Model file for the job. Use its own axes, mm. A direction names the side the tool comes from. Give positions to 0.01 mm unless a question says otherwise; leave off trailing zeros. Order: outer loops, then holes, each group sorted by start corner. A loop starts at its lowest first (then second) coordinate and runs counter-clockwise, first axis right, second up. Notation, with made-up numbers: (6, 35) - (10, 35) arc R6 cw to (10, 45) - close; hole circle Ø9 at (43.5, 52.5). An arc over 180 degrees is marked (long way). Use CSV: the item, a comma, the result in double quotes. Start each with the question number.
(1) Band-saw the part on B-B, the plane x = 0. Give the cut face in (y, z), then the cut area to 3 significant figures.
(2) Probe L1, parallel to Z at x = 5.2, y = 0 (3 decimals); L2, parallel to Z at x = 4, y = -1.25; L3, parallel to Y at x = 5.3, z = 7 (3 decimals). List the from-to ranges inside material, lowest first.
(3) Band-saw the part on C-C, the plane z = 11.5. Give the cut face in (x, y), then the cut area to 3 significant figures.
(4) Drop flat-ended pins along their axis: pin 1 Ø1 at (y, z) = (6, 15.5) entering from +X; pin 2 Ø10 at (y, z) = (-4, 25.5) entering from +X; pin 3 Ø8 at (x, z) = (-5, 24.5) entering from -Y; pin 4 Ø5 at (y, z) = (4, 29) entering from +X. Give the stop position or say it passes through.
(5) Pull direction X, two halves, no side cores. Call faces 1 (the cylindrical face through (4.57, -7.167, 16.769)), 2 (the cylindrical face through (-3.686, -0.162, 8.874)), 3 (the flat face through (3, 0, 34)): +X half, -X half, draft (parallel to the pull), parting line (faces both ways), or undercut.
(6) Band-saw the part on A-A, the plane y = 0. Give the cut face in (x, z) (3 decimals).
(7) Band-saw the part on D-D, the plane z = 27. Give the cut face in (x, y) (3 decimals), then the cut area to 3 significant figures.
(8) Tool access for faces 4 (the flat face through (1.815, 0, 29)), 5 (the flat face through (3.4, 1.9, 0)), 6 (the cylindrical face through (5.92, -1.36, 7.43)), 7 (the flat face through (0, 0, 18)): list every direction of +Z, -Z, +X, -X, +Y, -Y with a clear straight run to the whole face (end or side of a thin tool).
Autodesk Inventor part; units mm, degrees
ref_plane "Work Plane2" through (6, -1.3086, 34) normal (1, 0, 0) x (0, -1, 0)
ref_plane "YZ Plane" through (0, 0, 0) normal (1, 0, 0) x (0, 1, 0)
ref_plane "XZ Plane" through (0, 0, 0) normal (0, 1, 0) x (-1, 0, 0)
sketch "Sketch1" plane through (0, 0, 0) normal (0, 0, 1) x (1, 0, 0)
  circle A0 centre (0, 0) radius 8.5
  circle A1 centre (0, 0) radius 3.69
  dimension "d0" = 17
  dimension "d3" = 7.38
  dimension "d20" = 4.81
extrude "Extrusion2" add sketch "Sketch1" along normal blind 18
sketch "Sketch2" plane through (0, 0, 18) normal (0, 0, 1) x (1, 0, 0)
  circle A0 centre (0, 0) radius 8.5
  circle A1 centre (0, 0) radius 8.5
extrude "Extrusion3" add sketch "Sketch2" along normal blind 4
sketch "Sketch3" plane through (0, 0, 22) normal (0, 0, 1) x (1, 0, 0)
  arc A0 (1.815, 2.6173) -> (1.815, -2.6173) centre (0, 0) ccw
  circle A1 centre (0, 0) radius 8.5
  line L0 (1.815, 2.6173) -> (1.815, -2.6173)
  circle A2 centre (0, 0) radius 8.5
  dimension "d8" = 6.37
  dimension "d11" = 5
  dimension "d12" = 1.815
extrude "Extrusion4" add sketch "Sketch3" along normal blind 12
ref_plane "Work Plane2" through (6, -1.3086, 34) normal (1, 0, 0) x (0, -1, 0)
ref_plane "Work Plane1" through (1.815, -1.3086, 34) normal (1, 0, 0) x (0, -1, 0)
sketch "Sketch4" plane through (6, -1.3086, 34) normal (1, 0, 0) x (0, -1, 0)
  circle A0 centre (-1.3086, 7) radius 1.425
  circle A1 centre (-1.3086, 27) radius 1.425
  line L0 (-9.8086, 0) -> (7.1914, 0)
  line L1 (7.1914, 34) -> (-9.8086, 34)
  point P0 (-1.3086, 34)
  dimension "d14" = 2.85
  dimension "d15" = 7
  dimension "d16" = 7
extrude "Extrusion5" cut sketch "Sketch4" along normal blind 6.185 and the other way blind 5
fillet "Fillet1" radius 0.5 2 edges at (-8.5, 0, 34) (-8.5, 0, 0)
properties part number "schroefkoppeling motor en overbrening"
Answer block:
1,outline,"(-8.5, 0.5) arc R0.5 ccw to (-8, 0) - (-3.69, 0) - (-3.69, 18) - (3.69, 18) - (3.69, 0) - (8, 0) arc R0.5 ccw to (8.5, 0.5) - (8.5, 33.5) arc R0.5 ccw to (8, 34) - (3.19, 34) - (3.19, 22) - (-3.19, 22) - (-3.19, 34) - (-8, 34) arc R0.5 ccw to (-8.5, 33.5) - close"
1,area,"369 mm2"
2,L1,"z = 0 to 5.575, 8.425 to 25.575, 28.425 to 34"
2,L2,"z = 0 to 6.32, 7.68 to 26.32, 27.68 to 34"
2,L3,"y = -6.645 to -1.425, 1.425 to 6.645"
3,outline,"circle Ø17 at (0, 0); hole circle Ø7.38 at (0, 0)"
3,area,"184 mm2"
4,pin 1,"stops at x = 6.48"
4,pin 2,"stops at x = 8.5"
4,pin 3,"stops at y = -8.44"
4,pin 4,"stops at x = 8.37"
5,face 1,"parting line"
5,face 2,"undercut"
5,face 3,"draft"
6,outline,"(-8.5, 0.5) arc R0.5 ccw to (-8, 0) - (-3.69, 0) - (-3.69, 18) - (3.69, 18) - (3.69, 8.425) - (8.5, 8.425) - (8.5, 25.575) - (1.815, 25.575) - (1.815, 22) - (-3.185, 22) - (-3.185, 34) - (-8, 34) arc R0.5 ccw to (-8.5, 33.5) - close; (1.815, 28.425) - (8.5, 28.425) - (8.5, 33.5) arc R0.5 ccw to (8, 34) - (1.815, 34) - close; (3.69, 0) - (8, 0) arc R0.5 ccw to (8.5, 0.5) - (8.5, 5.575) - (3.69, 5.575) - close"
7,outline,"(1.815, -2.617) arc R3.185 cw (long way) to (1.815, 2.617) - (1.815, 1.425) - (8.38, 1.425) arc R8.5 ccw (long way) to (8.38, -1.425) - (1.815, -1.425) - close"
7,area,"181 mm2"
8,face 4,"+Z"
8,face 5,"-Z, +X, -X, +Y, -Y"
8,face 6,"+X"
8,face 7,"-Z"
